Input: part model. Units: mm. Frame: model coordinates. Face numbers are marked on the shaded views. A direction names the side the tool comes from. Coordinates: 2 decimals unless noted, no trailing zeros. Loops run counter-clockwise (first coordinate to the right, second up) from the corner with the lowest first, then second, coordinate; pieces in that order, holes last. Notation, with made-up numbers: (-29.5, 53.25) - (14.5, 53.25) arc R29 ccw to (14.5, 82.25) - close; hole circle Ø2 at (13, -15). An arc over 180 degrees is marked (long way). Write item = value, one per line. Start each with the question number.
from build123d import *

# Parameters (mm, degrees)
SKETCH_1_R          = 1.5
EXTRUDE_1_DEPTH     = 5
SKETCH_2_R          = 3
CUT_EXTRUDE_1_DEPTH = 10
SKETCH_3_R          = 4
SKETCH_3_R_2        = 3
EXTRUDE_1_2_DEPTH   = 4
CUT_EXTRUDE_START   = -4
CUT_EXTRUDE_2_DEPTH = 4


with BuildPart() as part:
    # 草图1 → Extrude 1 (new body)
    with BuildSketch(Plane.XY):
        with BuildLine():
            Line((-15.5, 27.5), (38.5, 27.5))
            ThreePointArc((38.5, 27.5), (40.621320344, 26.621320344), (41.5, 24.5))
            Line((41.5, 24.5), (41.5, -7))
            ThreePointArc((41.5, -7), (40.621320344, -9.121320344), (38.5, -10))
            Line((38.5, -10), (33.3, -10))
            Line((33.3, -10), (30.825, -10))
            Line((30.825, -10), (30.825, 10))
            Line((30.825, 10), (-9.175, 10))
            Line((-9.175, 10), (-9.175, -10))
            Line((-9.175, -10), (-15.5, -10))
            ThreePointArc((-15.5, -10), (-17.621320344, -9.121320344), (-18.5, -7))
            Line((-18.5, -7), (-18.5, 24.5))
            ThreePointArc((-18.5, 24.5), (-17.621320344, 26.621320344), (-15.5, 27.5))
        make_face()
        with Locations((-13.575, 5)):
            Circle(SKETCH_1_R, mode=Mode.SUBTRACT)
        with Locations((-13.575, -5)):
            Circle(SKETCH_1_R, mode=Mode.SUBTRACT)
        with Locations((35.025, 5)):
            Circle(SKETCH_1_R, mode=Mode.SUBTRACT)
        with Locations((35.025, -5)):
            Circle(SKETCH_1_R, mode=Mode.SUBTRACT)
    extrude(amount=EXTRUDE_1_DEPTH)

    # 草图2 → 切除-拉伸1 (cut)
    with BuildSketch(Plane.XY.offset(5)):
        with Locations((-6.17, 21.5)):
            Circle(SKETCH_2_R)
        with Locations((29.17, 21.5)):
            Circle(SKETCH_2_R)
    extrude(amount=-CUT_EXTRUDE_1_DEPTH, mode=Mode.SUBTRACT)

    # 草图3 → Extrude 1 2 (add)
    with BuildSketch(Plane.XY.offset(5)):
        with Locations((-8.5, 0)):
            Circle(SKETCH_3_R)
        with Locations((-8.5, 0)):
            Circle(SKETCH_3_R_2, mode=Mode.SUBTRACT)
    extrude(amount=EXTRUDE_1_2_DEPTH)

    # 草图5 → 切除-拉伸2 (cut)
    with BuildSketch(Plane.XY.offset(9).offset(CUT_EXTRUDE_START)):
        with BuildLine():
            Line((-6.115117964, 3.211282871), (-6.115117964, -3.211282871))
            ThreePointArc((-6.115117964, -3.211282871), (-4.5, 0), (-6.115117964, 3.211282871))
        make_face()
    extrude(amount=CUT_EXTRUDE_2_DEPTH, mode=Mode.SUBTRACT)


solid = part.part
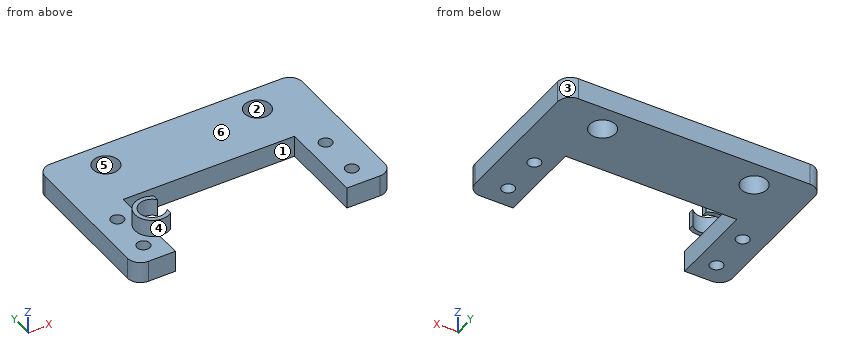
Item 1: Ray query, line 1 (X direction, y = -1.5, z = 1) (3 decimals); line 2 (Y direction, x = 10, z = 0.75); line 3 (X direction, y = -6, z = 3.75) (3 decimals). Return the intervals inside material, ascending.
Item 2: Cut plane B-B on x = 29.17. Return loops of the section in (y, z), plus the area to 3 significant figures.
Item 3: Pin query (flat end, axial travel): pin 1 (2.5 mm diameter, centred on x = -13.575, y = -5, fed in from -Z); pin 2 (3.5 mm diameter, centred on x = -8.5, y = 0, fed in from +Z); pin 3 (1.5 mm diameter, centred on x = -7.5, z = 1, fed in from -Y); pin 4 (0.7 mm diameter, centred on y = 2.5, z = 6.5, fed in from +X). Return the tip coordinate at first contact, or that it passes through.
Item 4: Access query for the marked faces 1 and 2. Directions: +Z, -Z, +X, -X, +Y, -Y. A direction counts if a zero-diameter tool reaches every point of the face in a straight line with its end or side. Return the directions, or none.
Item 5: Cut plane C-C on y = 5. Return loops of the section in (x, z) (3 decimals).
Item 6: Pull-direction query (X, two-part tool) for the marked faces 3, 4, 5 and 6; classes: pulls with the +X half, pulls with the -X half, needs draft (parallel to the pull), parting line crosses it, or undercut.
Item 7: Cut plane A-A on z = 1. Return loops of the section in (x, y) (3 decimals), plus the area to 3 significant figures.
Item 8: Cut plane D-D on y = 0. Return loops of the section in (x, z) (3 decimals).
Recorded:
q1.line_1 = -18.5 to -9.175, 30.825 to 41.5
q1.line_2 = 10 to 27.5
q1.line_3 = -18.5 to -14.693, -12.457 to -9.175, 30.825 to 33.907, 36.143 to 41.5
q2.outline = (10, 0) - (18.5, 0) - (18.5, 5) - (10, 5) - close; (24.5, 0) - (27.5, 0) - (27.5, 5) - (24.5, 5) - close
q2.area = 57.5 mm²
q3.pin_1 = through
q3.pin_2 = 5
q3.pin_3 = 10
q3.pin_4 = -6.12
q4.face_1 = +Z, -Z, -Y
q4.face_2 = +Z, -Z
q5.outline = (-18.5, 0) - (-15.075, 0) - (-15.075, 5) - (-18.5, 5) - close; (-12.075, 0) - (-9.175, 0) - (-9.175, 5) - (-12.075, 5) - close; (30.825, 0) - (33.525, 0) - (33.525, 5) - (30.825, 5) - close; (36.525, 0) - (41.5, 0) - (41.5, 5) - (36.525, 5) - close
q6.face_3 = pulls with the +X half
q6.face_4 = parting line crosses it
q6.face_5 = undercut
q6.face_6 = needs draft
q7.outline = (-18.5, -7) arc R3 ccw to (-15.5, -10) - (-9.175, -10) - (-9.175, 10) - (30.825, 10) - (30.825, -10) - (38.5, -10) arc R3 ccw to (41.5, -7) - (41.5, 24.5) arc R3 ccw to (38.5, 27.5) - (-15.5, 27.5) arc R3 ccw to (-18.5, 24.5) - close; hole circle Ø3 at (-13.575, -5); hole circle Ø3 at (-13.575, 5); hole circle Ø6 at (-6.17, 21.5); hole circle Ø6 at (29.17, 21.5); hole circle Ø3 at (35.025, -5); hole circle Ø3 at (35.025, 5)
q7.area = 1,360 mm²
q8.outline = (-18.5, 0) - (-9.175, 0) - (-9.175, 5) - (-11.5, 5) - (-11.5, 9) - (-12.5, 9) - (-12.5, 5) - (-18.5, 5) - close; (30.825, 0) - (41.5, 0) - (41.5, 5) - (30.825, 5) - close
